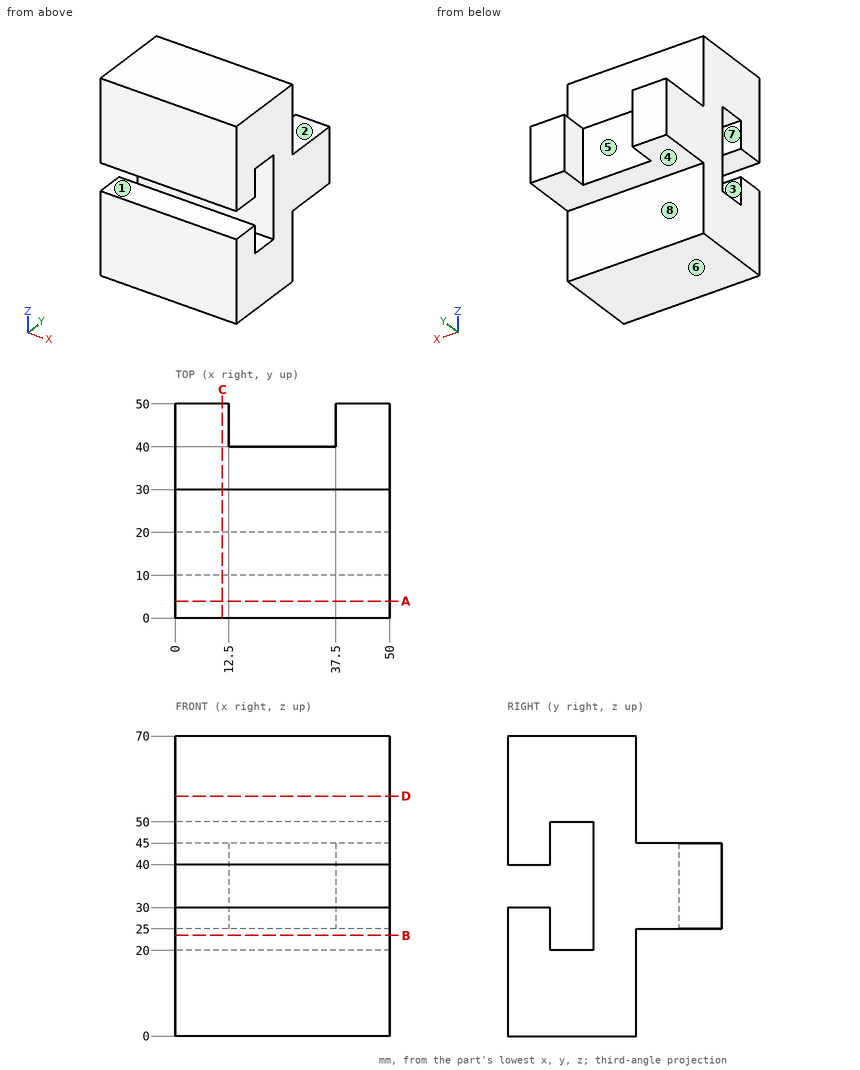
Here's the drawing with two shaded views (mm, measured from the low corner). I have some questions. A direction names the side the tool comes from. Give positions to 0.01 mm unless a question says otherwise; leave off trailing zeros. Write each loop counter-clockwise with the first axis right and the second up, starting at its lowest first coordinate (ties: lowest second). Pieces come first, ordered by that corner, then holes. Notation, with made-up numbers: (42.5, 13) -> (52.5, 13) arc R26 cw to (52.5, 41) -> close; hole circle Ø11 at (-38.75, 27.25). An arc over 180 degrees is marked (long way). Use one line per item in the form item = value. Start each with the question number.
1. On a 3-axis mill with a long thin cutter (end or side, diameter ignored), from which of +Z, -Z, +X, -X, +Y, -Y can I reach the whole of each face in a straight line? I mean the marked faces 1, 2, 3, 4 and 5. Say none if no direction works.
2. Thinking about a two-plate mould opening in Z: for the marked faces 6, 7 and 8, which applies, +Z half, -Z half, draft (parallel to the pull), parting line (faces both ways), or undercut?
3. Imagine slicing it at A-A on y = 4. List the corners of the cut face in (x, z) for me, plus the area to 3 significant figures.
4. If I drill on L1, parallel to Z at x = 42.5, y = 13; L2, parallel to X at y = 45, z = 44; L3, parallel to Z at x = 11.5, y = 5, over which ranges is the centre line in solid material (lowest first)?
5. Will these pins go through, and if not, where does the flat tip stop? pin 1 Ø10 at (x, z) = (20, 37) entering from +Y; pin 2 Ø5 at (x, y) = (7, 39.5) entering from -Z; pin 3 Ø1 at (x, y) = (17, 39) entering from +Z.
6. Imagine slicing it at B-B on z = 23.5. List the corners of the cut face in (x, y) for me.
7. Imagine slicing it at D-D on z = 56. List the corners of the cut face in (x, y) for me.
8. Imagine slicing it at C-C on x = 11. List the corners of the cut face in (y, z) for me.
Entries:
q1.face_1 = +X, -X, -Y
q1.face_2 = +Z, +X, -X, +Y
q1.face_3 = +X, -X
q1.face_4 = -Z, +X, -X, +Y
q1.face_5 = +Z, -Z, +Y
q2.face_6 = -Z half
q2.face_7 = undercut
q2.face_8 = draft
q3.outline = (0, 0) -> (50, 0) -> (50, 30) -> (0, 30) -> close; (0, 40) -> (50, 40) -> (50, 70) -> (0, 70) -> close
q3.area = 3,000 mm²
q4.L1 = 0 to 20, 50 to 70
q4.L2 = 0 to 12.5, 37.5 to 50
q4.L3 = 0 to 30, 40 to 70
q5.pin_1 = 40
q5.pin_2 = 25
q5.pin_3 = 45
q6.outline = (0, 0) -> (50, 0) -> (50, 10) -> (0, 10) -> close; (0, 20) -> (50, 20) -> (50, 30) -> (0, 30) -> close
q7.outline = (0, 0) -> (50, 0) -> (50, 30) -> (0, 30) -> close
q8.outline = (0, 0) -> (30, 0) -> (30, 25) -> (50, 25) -> (50, 45) -> (30, 45) -> (30, 70) -> (0, 70) -> (0, 40) -> (10, 40) -> (10, 50) -> (20, 50) -> (20, 20) -> (10, 20) -> (10, 30) -> (0, 30) -> close
